Could you check a few things on this model? Use its own coordinates, in mm. A direction names the side the tool comes from. Give positions to 0.01 mm unless a question says otherwise; leave off trailing zeros. Write each loop counter-clockwise with the first axis right and the second up, starting at its lowest first coordinate (ties: lowest second). Pieces come first, ordered by that corner, then holes. Notation, with made-up numbers: (47.5, 33.5) - (92.5, 33.5) arc R35 cw to (92.5, 65.5) - close; hole circle Ø7 at (41, 22.5). An arc over 180 degrees is marked (long way). Write item = value, one per line.
from build123d import *

# Parameters (mm, degrees)
SKETCH1_R               = 2
BOSS_EXTRUDE1_DEPTH     = 4
FILLET10_R              = 1
FILLET11_R              = 10
FILLET12_R              = 5
FILLET13_R              = 5
FILLET14_R              = 5
SKETCH2_R               = 2
CUT_EXTRUDE1_DEPTH      = 20
CUT_EXTRUDE2_DEPTH      = 0.5
FILLET15_R              = 10
CUT_EXTRUDE3_DEPTH      = 97.958369289
CUT_EXTRUDE3_DEPTH_BACK = 97.958369289
FILLET15_OF_MIRROR1_R   = 10


with BuildPart() as part:
    # Sketch1 → Boss-Extrude1 (new body)
    with BuildSketch(Plane.XY):
        with BuildLine():
            Line((-5, -5), (-5, 46.428571429))
            ThreePointArc((-5, 46.428571429), (5.360662074, 77.221028176), (35.086282243, 90.332329282))
            Line((35.086282243, 90.332329282), (35.086282243, 80.08008038))
            ThreePointArc((35.086282243, 80.08008038), (5.086282243, 50.08008038), (35.086282243, 20.08008038))
            Line((35.086282243, 20.08008038), (35.086282243, 14.08008038))
            ThreePointArc((35.086282243, 14.08008038), (31.017062028, 14.31079961), (27, 15))
            Line((27, 15), (27, -5))
            Line((27, -5), (-5, -5))
        make_face()
        Circle(SKETCH1_R, mode=Mode.SUBTRACT)
        with Locations((18, 0)):
            Circle(SKETCH1_R, mode=Mode.SUBTRACT)
    extrude(amount=BOSS_EXTRUDE1_DEPTH)

    # Fillet10
    fillet10_edges = [part.edges().sort_by_distance(p)[0] for p in [
        (35.086282243, 90.332329282, 2),
        (35.086282243, 80.08008038, 2),
        (35.086282243, 20.08008038, 2),
        (35.086282243, 14.08008038, 2),
    ]]
    fillet(fillet10_edges, radius=FILLET10_R)

    # Fillet11
    # the kernel refuses this fillet: 10 mm, written as the material it adds along each edge
    with BuildSketch(Plane(origin=(-5, 46.428571429, 0), x_dir=(-0.08596186737445177, 0.996298427860597, 0), z_dir=(0, 0, 1))) as fillet11_piece_1:
        with BuildLine():
            CenterArc((0.431926178, 9.999886119), FILLET11_R, 265.068661729, 4.657897264)
            Line((-0.427692496, 0.03690184), (0, 0))
            ThreePointArc((0, 0), (0.19210095, 0.000458397), (0.3842019, 0))
        make_face()
    extrude(amount=4)

    # Fillet12
    fillet12_edges = [part.edges().sort_by_distance(p)[0] for p in [
        (-5, -5, 2),
    ]]
    fillet(fillet12_edges, radius=FILLET12_R)

    # Fillet13
    fillet13_edges = [part.edges().sort_by_distance(p)[0] for p in [
        (27, -5, 2),
    ]]
    fillet(fillet13_edges, radius=FILLET13_R)

    # Fillet14
    fillet14_edges = [part.edges().sort_by_distance(p)[0] for p in [
        (27, 15, 2),
    ]]
    fillet(fillet14_edges, radius=FILLET14_R)

    # Sketch2 → Cut-Extrude1 (cut)
    with BuildSketch(Plane.XY.offset(4)):
        with Locations((10.086282243, 74.574977808)):
            Circle(SKETCH2_R)
        with Locations((11.117766586, 24.574977808)):
            Circle(SKETCH2_R)
    extrude(amount=-CUT_EXTRUDE1_DEPTH, mode=Mode.SUBTRACT)

    # Sketch3 → Cut-Extrude2 (cut)
    with BuildSketch(Plane(origin=(0, 0, 0), x_dir=(-1, 0, 0), z_dir=(0, 0, -1))):
        with BuildLine():
            Line((-14.777268977, -5), (-14.777268977, 7.317916248))
            Line((-14.777268977, 7.317916248), (-4.032042708, 20.652353666))
            Line((-4.032042708, 20.652353666), (-10.590052553, 32.761456562))
            ThreePointArc((-10.590052553, 32.761456562), (-9.00780857, 35.250609355), (-7.677638466, 37.883103447))
            Line((-7.677638466, 37.883103447), (1.949636164, 20.106725877))
            Line((1.949636164, 20.106725877), (-9.777268977, 5.554060462))
            Line((-9.777268977, 5.554060462), (-9.777268977, -5))
            Line((-9.777268977, -5), (-14.777268977, -5))
        make_face()
    cut_extrude2 = extrude(amount=-CUT_EXTRUDE2_DEPTH, mode=Mode.SUBTRACT)

    # Fillet15
    fillet15_edges = [part.edges().sort_by_distance(p)[0] for p in [
        (14.777268977, 7.317916248, 0.25),
        (4.032042708, 20.652353666, 0.25),
        (-1.949636164, 20.106725877, 0.25),
        (9.777268977, 5.554060462, 0.25),
    ]]
    fillet(fillet15_edges, radius=FILLET15_R)

    # Sketch4 → Cut-Extrude3 (cut, two sides: drawn at the far end of the back side and taken through both)
    with BuildSketch(Plane(origin=(0, 0, 0.5), x_dir=(-1, 0, 0), z_dir=(0, 0, -1)).offset(-CUT_EXTRUDE3_DEPTH_BACK)):
        with BuildLine():
            Line((-10.590052553, 32.761456562), (-8.89610131, 29.63364334))
            Line((-8.89610131, 29.63364334), (-5.738375915, 34.302332705))
            Line((-5.738375915, 34.302332705), (-7.677638466, 37.883103447))
            ThreePointArc((-7.677638466, 37.883103447), (-9.00780857, 35.250609355), (-10.590052553, 32.761456562))
        make_face()
    extrude(amount=CUT_EXTRUDE3_DEPTH + CUT_EXTRUDE3_DEPTH_BACK, mode=Mode.SUBTRACT)

    # Mirror1: Cut-Extrude2 across plane
    add(cut_extrude2.mirror(Plane.XY.offset(2)), mode=Mode.SUBTRACT)

    # Fillet15 of Mirror1
    fillet15_of_mirror1_edges = [part.edges().sort_by_distance(p)[0] for p in [
        (14.777268977, 7.317916248, 3.75),
        (4.032042708, 20.652353666, 3.75),
        (-1.949636164, 20.106725877, 3.75),
        (9.777268977, 5.554060462, 3.75),
    ]]
    fillet(fillet15_of_mirror1_edges, radius=FILLET15_OF_MIRROR1_R)


solid = part.part
1. Thinking about a two-plate mould opening in Y: for faces 1 (the face through (27, 5, 2)), 2 (the face through (7.339, 31.935, 2.021)), 3 (the face through (11, -5, 2)), which applies, pulls with the +Y half, pulls with the -Y half, needs draft (parallel to the pull), parting line crosses it, or undercut?
Filled sheet:
face_1 = needs draft
face_2 = undercut
face_3 = pulls with the -Y half
2. If we section it at A-A, the plane x = 18: Please give me the cut outline in (y, z), and give its area (3 significant figures).
Filled sheet:
outline = (-5, 0) - (-2, 0) - (-2, 4) - (-5, 4) - close; (2, 0) - (25.42, 0) - (25.42, 4) - (2, 4) - close; (74.74, 0) - (86.53, 0) - (86.53, 4) - (74.74, 4) - close
area = 153 mm2
3. If we section it at D-D, the plane x = -1: Please give me the cut outline in (y, z), and give its area (3 significant figures).
Filled sheet:
outline = (-4.9, 0) - (-1.73, 0) - (-1.73, 4) - (-4.9, 4) - close; (1.73, 0) - (67.91, 0) - (67.91, 4) - (1.73, 4) - close
area = 277 mm2
4. For pin 1 (0.6 mm diameter, centred on y = 0, z = 3.5, fed in from +X); pin 2 (1 mm diameter, centred on y = 58, z = 2.5, fed in from +X); pin 3 (2 mm diameter, centred on y = 13.5, z = 2, fed in from -X), each with a flat end and sliding along its axis, tell me the tip position at first contact or that it passes through.
Filled sheet:
pin_1 = 27
pin_2 = 6.29
pin_3 = -5
5. If we section it at B-B, the plane z = 2.25: Please give me the cut outline in (x, y), and give its area (3 significant figures).
Filled sheet:
outline = (-5.03, 46.81) arc R10 cw to (-5, 46) - (-5, 0) arc R5 ccw to (0, -5) - (22, -5) arc R5 ccw to (27, 0) - (27, 9.2) arc R5 cw to (32.38, 14.18) arc R36 ccw to (34.06, 14.09) arc R1 ccw to (35.09, 15.09) - (35.09, 19.1) arc R1 ccw to (34.12, 20.1) arc R30 cw to (10.59, 32.76) - (8.9, 29.63) - (5.74, 34.3) - (7.68, 37.88) arc R30 cw to (34.12, 80.06) arc R1 ccw to (35.09, 81.06) - (35.09, 89.32) arc R1 ccw to (34.06, 90.32) arc R40.25 ccw to start; hole circle Ø4 at (0, 0); hole circle Ø4 at (10.09, 74.57); hole circle Ø4 at (11.12, 24.57); hole circle Ø4 at (18, 0)
area = 1,840 mm2
6. If we section it at C-C, the plane x = 23.5: Please give me the cut outline in (y, z), and give its area (3 significant figures).
Filled sheet:
outline = (-4.77, 0) - (22.41, 0) - (22.41, 4) - (-4.77, 4) - close; (77.75, 0) - (88.63, 0) - (88.63, 4) - (77.75, 4) - close
area = 152 mm2
7. I need wall thicknesses on line 1 (Y direction, x = 18, z = 2.65); line 2 (X direction, y = 8, z = 2.8); line 3 (Y direction, x = 21, z = 1.7). Which ranges of each line are inside material? Lowest first, please.
Filled sheet:
line_1 = -5 to -2, 2 to 25.42, 74.74 to 86.53
line_2 = -5 to 27
line_3 = -5 to 23.59, 76.57 to 87.79
8. Which directions (+Z, -Z, +X, -X, +Y, -Y) give clear straight access to the entire face, cutting with the end or side of a thin tool? Please do faces 4 (the face through (14.192, 7.162, 0.254)), 5 (the face through (9.223, 5.308, 0.254)), 6 (the face through (6.045, 20.753, 3.746)).
Filled sheet:
face_4 = -Z, -Y
face_5 = -Z
face_6 = +Z
